The model under review builds one solid part; all positions refer to its coordinate system, in mm. A direction names the side the tool comes from. Coordinates: 2 decimals unless noted, no trailing zeros. Order: outer loops, then holes, each group sorted by start corner. A loop starts at its lowest first (then second) coordinate and runs counter-clockwise, first axis right, second up. Notation, with made-up numbers: M 21.5,41 L 73.5,41 A24 cw 73.5,64 Z; hole C -17,-31 d3. An arc over 180 degrees is marked long. Answer in a Markdown table with one row per item.
Autodesk Inventor part; units mm, degrees
ref_plane "YZ Plane" through (0, 0, 0) normal (1, 0, 0) x (0, 1, 0)
ref_plane "XZ Plane" through (0, 0, 0) normal (0, 1, 0) x (-1, 0, 0)
ref_plane "XY Plane" through (0, 0, 0) normal (0, 0, 1) x (1, 0, 0)
sketch "Sketch1" plane through (0, 0, 0) normal (0, 1, 0) x (-1, 0, 0)
  line L0 (-35, 10) -> (-40.1, 10)
  line L1 (-40.1, 10) -> (-40.1, -50)
  line L2 (-40.1, -50) -> (-35.1, -50)
  line L3 (-35, 5) -> (-32, 5)
  line L4 (-32, 5) -> (-32, -10)
  line L5 (-32, -10) -> (-23, -10)
  line L6 (-23, -11) -> (-23, -15.9282)
  line L7 (-22, -16.9282) -> (-27, -16.9282)
  line L8 (-27, -16.9282) -> (-27, -21.9282)
  line L9 (-27, -21.9282) -> (-21.8, -21.9282)
  line L10 (-21.8, -21.9282) -> (-21.8, -24.9282)
  line L11 (-21.8, -24.9282) -> (-27, -24.9282)
  line L12 (-27, -24.9282) -> (-27, -29.9282)
  line L13 (-27, -29.9282) -> (-21.8, -29.9282)
  line L14 (-21.8, -29.9282) -> (-21.8, -32.9282)
  line L15 (-21.8, -32.9282) -> (-27, -32.9282)
  line L16 (-27, -32.9282) -> (-27, -37.9282)
  line L17 (-27, -37.9282) -> (-21.8, -37.9282)
  line L18 (-21.8, -37.9282) -> (-21.8, -40.9282)
  line L19 (-21.8, -40.9282) -> (-28, -40.9282)
  line L20 (-23, -10) -> (-21, -10)
  line L21 (-21, -10) -> (-21, -11)
  line L22 (-21, -11) -> (-23, -11)
  line L23 (-22, -16.9282) -> (-21, -16.9282)
  line L24 (-21, -16.9282) -> (-21, -15.9282)
  line L25 (-21, -15.9282) -> (-23, -15.9282)
  line L26 (-28, -40.9282) -> (-28, -50)
  line L27 (-28, -50) -> (-35.1, -50)
  line L28 (-35, 5) -> (-35, 10)
  line L29 (0, -62) -> (0, 22)
  point P0 (0, 0)
  point P1 (-33.5, 5)
  dimension "d4" = 3
  dimension "d6" = 23
  dimension "d7" = 5
  dimension "d8" = 5
  dimension "d11" = 3
  dimension "d12" = 5
  dimension "d13" = 3
  dimension "d14" = 5
  dimension "d15" = 3
  dimension "d16" = 2
  dimension "d17" = 1
  dimension "d18" = 1
  dimension "d19" = 28
  dimension "d20" = 27
  dimension "d21" = 27
  dimension "d22" = 23
  dimension "d28" = 15
  dimension "d29" = 5
  dimension "d30" = 32
revolve "Revolution1" add sketch "Sketch1" angle 360 about axis through (0, 0, -10) along (0, 0, 1)
sketch "Sketch2" plane through (0, 0, 10) normal (0, 0, 1) x (1, 0, 0)
  line L0 (-41.9384, 10) -> (42.6332, 10)
  line L1 (42.6332, 10) -> (42.6332, 41.1939)
  line L2 (42.6332, 41.1939) -> (-41.9384, 41.1939)
  line L3 (-41.9384, 41.1939) -> (-41.9384, 10)
  point P0 (0, 0)
extrude "Extrusion1" cut sketch "Sketch2" against normal through all
sketch "Sketch3" plane through (0, 0, -10) normal (0, 0, 1) x (1, 0, 0)
  arc A0 (-25.0799, 10) -> (25.0799, 10) centre (0, 0) ccw
  line L0 (-27, 0) -> (27, 0)
  line L1 (27, 0) -> (27, 40.4991)
  line L2 (27, 40.4991) -> (-27, 40.4991)
  line L3 (-27, 40.4991) -> (-27, 0)
extrude "Extrusion2" cut sketch "Sketch3" against normal through all contours L3 L2 L1 L0
sketch "Sketch4" plane through (0, 0, 10) normal (0, 0, 1) x (1, 0, 0)
  arc A0 (-38.8331, 10) -> (38.8331, 10) centre (0, 0) ccw
  line L0 (12.5184, -42.1041) -> (-12.5184, -42.1041)
  line L1 (-12.5184, -42.1041) -> (-12.5184, -38.0959)
  line L2 (-12.5184, -38.0959) -> (12.5184, -38.0959)
  line L3 (12.5184, -38.0959) -> (12.5184, -42.1041)
  line L4 (12.5184, -42.1041) -> (-12.5184, -38.0959) construction
  line L5 (-12.5184, -42.1041) -> (12.5184, -38.0959) construction
  point P0 (0, -40.1)
extrude "Extrusion3" add sketch "Sketch4" against normal up to surface (60 mm away)
properties part number "HAL-filter-holder1"
(1) Machinability: for faces 4 (the flat face through (-12.518, -40, -20)), 5 (the flat face through (-4, -21, -11)), 6 (the cylindrical face through (0.479, -21.795, -39.449)), which of the approach directions +Z, -Z, +X, -X, +Y, -Y give a long, thin tool a straight path to every point of the face, cutting with its end or side? Answer none if there is none.
Report:
| item | result |
|---|---|
| face 4 | +Z, -Z, -X, -Y |
| face 5 | +Y |
| face 6 | -Z, +Y |
(2) Take a section at A-A (z = -31). Write out the cut boundary in (x, y).
Report:
| item | result |
|---|---|
| outline | M -38.83,10 A40.1 ccw -12.52,-38.1 L -12.52,-42.1 L 12.52,-42.1 L 12.52,-38.1 A40.1 ccw 38.83,10 L 27,10 L 27,0 L 21.8,0 A21.8 cw -21.8,0 L -27,0 L -27,10 Z |
(3) Take a section at C-C (x = 0). Write out the cut boundary in (y, z).
Report:
| item | result |
|---|---|
| outline | M -42.1,-50 L -28,-50 L -28,-40.93 L -21.8,-40.93 L -21.8,-37.93 L -27,-37.93 L -27,-32.93 L -21.8,-32.93 L -21.8,-29.93 L -27,-29.93 L -27,-24.93 L -21.8,-24.93 L -21.8,-21.93 L -27,-21.93 L -27,-16.93 L -21,-16.93 L -21,-15.93 L -23,-15.93 L -23,-11 L -21,-11 L -21,-10 L -32,-10 L -32,5 L -35,5 L -35,10 L -42.1,10 Z |
(4) Insertion check: P1, Ø2, axis at x = 6, y = -24, coming from the -Z side; P2, Ø0.9, axis at x = -23, z = -39, coming from the +Y side; P3, Ø22.5, axis at x = -7.5, y = -22.5, coming from the +Z side. Each pin has a flat end and moves straight along its axis. Give the tip position at first contact, or say it passes through.
Report:
| item | result |
|---|---|
| P1 | z = -40.93 |
| P2 | y = 0 |
| P3 | z = 5 |
(5) Take a section at B-B (y = 4.5). Write out the cut boundary in (x, z), then the cut area to 3 significant figures.
Report:
| item | result |
|---|---|
| outline | M -39.85,-50 L -27.64,-50 L -27.64,-40.93 L -27,-40.93 L -27,-10 L -31.68,-10 L -31.68,5 L -34.71,5 L -34.71,10 L -39.85,10 Z; M 27,-40.93 L 27.64,-40.93 L 27.64,-50 L 39.85,-50 L 39.85,10 L 34.71,10 L 34.71,5 L 31.68,5 L 31.68,-10 L 27,-10 Z |
| area | 1,310 mm^2 |
(6) The part is to be moulded in two halves that separate along Y. For faces 1 (the flat face through (0, -22, -32.928)), 2 (the cylindrical face through (0.85, -31.99, -2.61)), 3 (the cylindrical face through (-0.462, -20.995, -16.421)), say which applies: +Y half, -Y half, draft (parallel to the pull), parting line (faces both ways), or undercut.
Report:
| item | result |
|---|---|
| face 1 | draft |
| face 2 | undercut |
| face 3 | +Y half |
(7) Take a section at D-D (z = -19). Write out the cut boundary in (x, y).
Report:
| item | result |
|---|---|
| outline | M -38.83,10 A40.1 ccw -12.52,-38.1 L -12.52,-42.1 L 12.52,-42.1 L 12.52,-38.1 A40.1 ccw 38.83,10 L 27,10 L 27,0 A27 cw -27,0 L -27,10 Z |
(8) To check wall thickness, follow line 1 (X direction, y = 0, z = -44.5); line 2 (Z direction, x = 1, y = -24); line 3 (X direction, y = 0, z = 7.1). State the ranges of each line that lie inside material, in increasing order. Write a range as [from, to].
Report:
| item | result |
|---|---|
| line 1 | [-40.1, -28], [28, 40.1] |
| line 2 | [-40.93, -37.93], [-32.93, -29.93], [-24.93, -21.93], [-16.93, -10] |
| line 3 | [-40.1, -35], [35, 40.1] |
